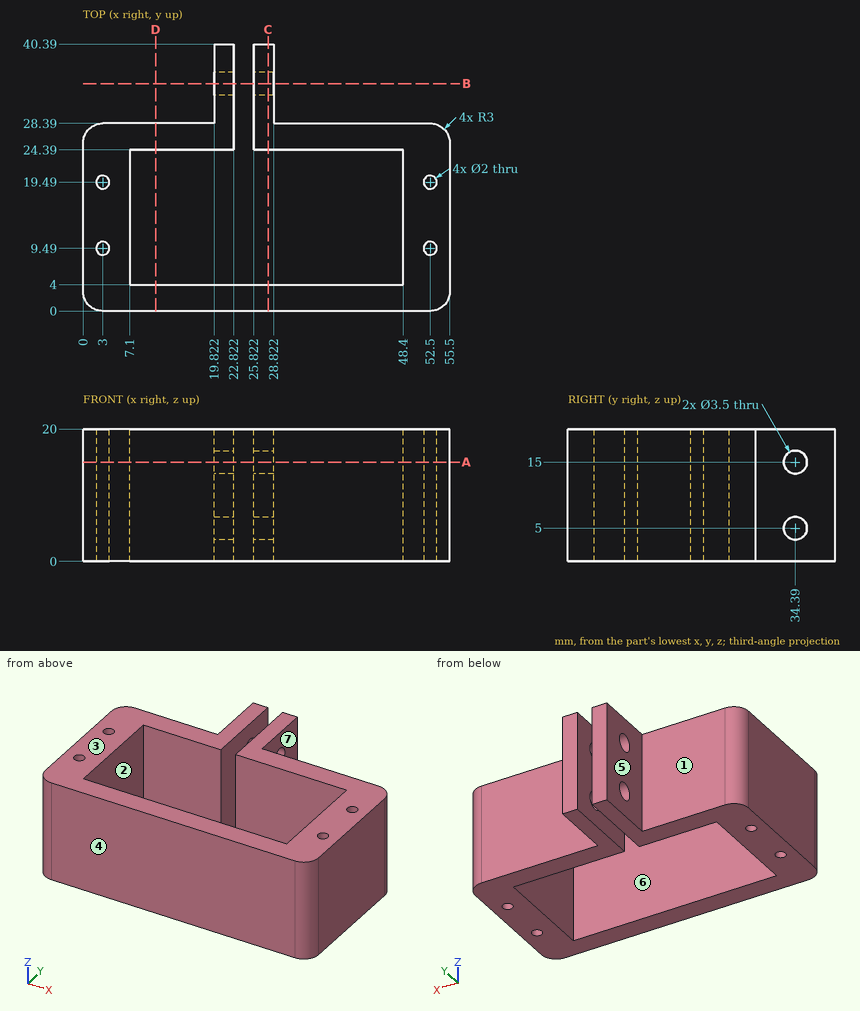
The drawing under review shows one solid part. Ordinate dimensions are in mm from its lowest x, y, z. A direction names the side the tool comes from. Round coordinates to 2 decimals unless told otherwise and drop trailing zeros. Order: outer loops, then holes, each group sorted by start corner. A loop starts at its lowest first (then second) coordinate and runs counter-clockwise, first axis right, second up. Notation, with made-up numbers: (-6, 50) - (36, 50) arc R20 cw to (36, 80) - close; hole circle Ø11 at (35, 32.5). An arc over 180 degrees is marked (long way). Return JSON: item names as keys, results as strings.
Q1. Consider section C-C on x = 28. Write out the cut boundary in (y, z), plus the area to 3 significant figures.
Computed values:
{"outline": "(0, 0) - (4, 0) - (4, 20) - (0, 20) - close; (24.39, 0) - (40.39, 0) - (40.39, 20) - (24.39, 20) - close; hole circle Ø3.5 at (34.39, 5); hole circle Ø3.5 at (34.39, 15)", "area": "381 mm2"}
Q2. Consider section B-B on y = 34.39. Write out the cut boundary in (x, z), plus the area to 3 significant figures.
Computed values:
{"outline": "(19.82, 0) - (22.82, 0) - (22.82, 3.25) - (19.82, 3.25) - close; (19.82, 6.75) - (22.82, 6.75) - (22.82, 13.25) - (19.82, 13.25) - close; (19.82, 16.75) - (22.82, 16.75) - (22.82, 20) - (19.82, 20) - close; (25.82, 0) - (28.82, 0) - (28.82, 3.25) - (25.82, 3.25) - close; (25.82, 6.75) - (28.82, 6.75) - (28.82, 13.25) - (25.82, 13.25) - close; (25.82, 16.75) - (28.82, 16.75) - (28.82, 20) - (25.82, 20) - close", "area": "78.0 mm2"}
Q3. Consider section D-D on x = 11. Write out the cut boundary in (y, z), plus the area to 3 significant figures.
Computed values:
{"outline": "(0, 0) - (4, 0) - (4, 20) - (0, 20) - close; (24.39, 0) - (28.39, 0) - (28.39, 20) - (24.39, 20) - close", "area": "160 mm2"}
Q4. Consider section A-A on z = 15. Give the number of separate pieces and of enclosed holes in the cut face, plus the area to 3 significant figures.
Computed values:
{"separate pieces": "3", "enclosed holes": "4", "area": "752 mm2"}
Q5. Machinability: for the marked faces 4, 5, 6 and 7, which of the approach directions +Z, -Z, +X, -X, +Y, -Y give a long, thin tool a straight path to every point of the face, cutting with its end or side? Answer none if there is none.
Computed values:
{"face 4": "+Z, -Z, +X, -X, -Y", "face 5": "+Z, -Z, -X, +Y", "face 6": "+Z, -Z", "face 7": "+Z, -Z, +X, +Y"}
Q6. For pin 1 Ø5 at (y, z) = (28.5, 9.5) entering from -X; pin 2 Ø4.5 at (y, z) = (34.39, 5) entering from +X; pin 3 Ø2 at (y, z) = (34.39, 15) entering from -X; pin 4 Ø8 at (y, z) = (31.5, 6.5) entering from -X, all flat-tipped, find the tip position at first contact; note any pin that passes through.
Computed values:
{"pin 1": "stops at x = 0.06", "pin 2": "stops at x = 28.82", "pin 3": "passes through", "pin 4": "stops at x = 0.87"}
Q7. The part is to be moulded in two halves that separate along Y. For the marked faces 1, 2 and 3, say which applies: pulls with the +Y half, pulls with the -Y half, needs draft (parallel to the pull), parting line crosses it, or undercut.
Computed values:
{"face 1": "pulls with the +Y half", "face 2": "undercut", "face 3": "needs draft"}
Q8. Wall thickness on L1, parallel to Z at x = 20.8, y = 34.39; L2, parallel to Y at x = 3, z = 4.5; L3, parallel to Y at x = 28.15, z = 5: over which ranges is each line inside the solid? List them lowest first. Write a range as [from, to].
Computed values:
{"L1": "z = [0, 3.25], [6.75, 13.25], [16.75, 20]", "L2": "y = [0, 8.49], [10.49, 18.49], [20.49, 28.39]", "L3": "y = [0, 4], [24.39, 32.64], [36.14, 40.39]"}
